```python
from build123d import *
from build123d.topology import SkipClean

# Parameters (mm, degrees)
SKETCH2_R           = 85
SKETCH2_R_2         = 20
BOSS_EXTRUDE1_DEPTH = 5
BOSS_EXTRUDE2_START = 155
SKETCH3_W           = 245
SKETCH3_H           = 230
SKETCH3_R           = 85
SKETCH3_W_2         = 265
SKETCH3_H_2         = 285
SKETCH3_R_2         = 20
BOSS_EXTRUDE2_DEPTH = 155
SKETCH4_W           = 33
SKETCH4_H           = 40
BOSS_EXTRUDE4_DEPTH = 70
SKETCH6_R           = 15
SKETCH6_W           = 63
SKETCH6_H           = 50
BOSS_EXTRUDE6_DEPTH = 22
SKETCH6_3_R         = 15
SKETCH6_3_R_2       = 6
BOSS_EXTRUDE7_DEPTH = 47
SKETCH6_4_R         = 6
BOSS_EXTRUDE8_DEPTH = 77
SKETCH2_4_R         = 85
CUT_EXTRUDE2_DEPTH  = 5


with BuildPart() as part:
    # Sketch2 → Boss-Extrude1 (new body)
    with BuildSketch(Plane.XY):
        Circle(SKETCH2_R)
        Circle(SKETCH2_R_2, mode=Mode.SUBTRACT)
    extrude(amount=BOSS_EXTRUDE1_DEPTH)

    # Sketch3 → Boss-Extrude2 (add)
    # profile 1 of 3: a face of its own
    with SkipClean():  # the faces are left unmerged after this step: merging them gives an invalid solid
        with BuildSketch(Plane(origin=(0, 0, 0), x_dir=(-1, 0, 0), z_dir=(0, 0, -1)).offset(BOSS_EXTRUDE2_START)):
            with Locations((-17.5, -20)):
                Rectangle(SKETCH3_W, SKETCH3_H)
            with Locations(Location((0, 0, 0), (0, 0, 180))):
                Circle(SKETCH3_R, mode=Mode.SUBTRACT)
        # profile 2 of 3: a face of its own
        with BuildSketch(Plane(origin=(0, 0, 0), x_dir=(-1, 0, 0), z_dir=(0, 0, -1)).offset(BOSS_EXTRUDE2_START)):
            with Locations((-272.5, 7.5)):
                Rectangle(SKETCH3_W_2, SKETCH3_H_2)
        # profile 3 of 3: a face of its own
        with BuildSketch(Plane(origin=(0, 0, 0), x_dir=(-1, 0, 0), z_dir=(0, 0, -1)).offset(BOSS_EXTRUDE2_START)):
            with Locations(Location((0, 0, 0), (0, 0, 180))):
                Circle(SKETCH3_R)
            Circle(SKETCH3_R_2, mode=Mode.SUBTRACT)
        extrude(amount=-BOSS_EXTRUDE2_DEPTH)

    # Sketch4 → Boss-Extrude4 (add)
    with SkipClean():  # the faces are left unmerged after this step: merging them gives an invalid solid
        with BuildSketch(Plane(origin=(0, 0, -155), x_dir=(-1, 0, 0), z_dir=(0, 0, -1))):
            with Locations((-83.5, 115)):
                Rectangle(SKETCH4_W, SKETCH4_H)
        extrude(amount=-BOSS_EXTRUDE4_DEPTH)

    # Sketch6 → Boss-Extrude6 (add)
    # profile 1 of 2: a face of its own
    with SkipClean():  # the faces are left unmerged after this step: merging them gives an invalid solid
        with BuildSketch(Plane.XZ.offset(135)):
            Polygon((-115, 50), (-115, 0), (-105, 0), (-52, 0), (-52, 50), align=None)
            with Locations(Location((-83.5, 25, 0), (0, 0, 270))):
                Circle(SKETCH6_R, mode=Mode.SUBTRACT)
        # profile 2 of 2: a face of its own
        with BuildSketch(Plane.XZ.offset(135)):
            with Locations((83.5, 25)):
                Rectangle(SKETCH6_W, SKETCH6_H)
            with Locations(Location((83.5, 25, 0), (0, 0, 270))):
                Circle(SKETCH6_R, mode=Mode.SUBTRACT)
        extrude(amount=-BOSS_EXTRUDE6_DEPTH)

    # Sketch6<3> → Boss-Extrude7 (add)
    # profile 1 of 2: a face of its own
    with SkipClean():  # the faces are left unmerged after this step: merging them gives an invalid solid
        with BuildSketch(Plane.XZ.offset(135)):
            with Locations(Location((-83.5, 25, 0), (0, 0, 270))):
                Circle(SKETCH6_3_R)
            with Locations(Location((-83.5, 25, 0), (0, 0, 270))):
                Circle(SKETCH6_3_R_2, mode=Mode.SUBTRACT)
        # profile 2 of 2: a face of its own
        with BuildSketch(Plane.XZ.offset(135)):
            with Locations(Location((83.5, 25, 0), (0, 0, 270))):
                Circle(SKETCH6_3_R)
            with Locations(Location((83.5, 25, 0), (0, 0, 270))):
                Circle(SKETCH6_3_R_2, mode=Mode.SUBTRACT)
        extrude(amount=-BOSS_EXTRUDE7_DEPTH)

    # Sketch6<4> → Boss-Extrude8 (add)
    with SkipClean():  # the faces are left unmerged after this step: merging them gives an invalid solid
        with BuildSketch(Plane.XZ.offset(135)):
            with Locations(Location((-83.5, 25, 0), (0, 0, 270))):
                Circle(SKETCH6_4_R)
            with Locations(Location((83.5, 25, 0), (0, 0, 270))):
                Circle(SKETCH6_4_R)
        extrude(amount=-BOSS_EXTRUDE8_DEPTH)

    # Sketch2<4> → Cut-Extrude2 (cut)
    with BuildSketch(Plane.XY):
        Circle(SKETCH2_4_R)
    extrude(amount=CUT_EXTRUDE2_DEPTH, mode=Mode.SUBTRACT)


solid = part.part
```
Here's how the part is built. I have some questions about the finished solid (model axes, mm). A direction names the side the tool comes from. Give positions to 0.01 mm unless a question says otherwise; leave off trailing zeros. Loops run counter-clockwise (first coordinate to the right, second up) from the corner with the lowest first, then second, coordinate; pieces in that order, holes last. Notation, with made-up numbers: M 36.25,-38 L 43.25,-38 A21 cw 43.25,0 Z; hole C 70,83 d7. An arc over 180 degrees is marked long. Use one line per item in the form item = value. Start each with the question number.
Q1. Will these pins go through, and if not, where does the flat tip stop? pin 1 Ø6 at (x, y) = (187, 96) entering from +Z; pin 2 Ø3 at (x, y) = (-108, -128.5) entering from -Z; pin 3 Ø16.5 at (x, y) = (83, 113.5) entering from +Z.
Q2. If we section it at B-B (y = 0): Write out the boundary of the cut face in (x, z).
Q3. If we section it at A-A (z = -126.5): Write out the boundary of the cut face in (x, y).
Q4. Thinking about a two-plate mould opening in Z: for faces 1 (the flat face through (154, 9, -155)), 2 (the flat face through (-83.3, -88, 18.5)), 3 (the flat face through (405, 6, -79)), 4 (the flat face through (84, 115, -85)), which applies, +Z half, -Z half, draft (parallel to the pull), parting line (faces both ways), or undercut?
Q5. If we section it at C-C (x = -83.5): Write out the boundary of the cut face in (y, z).
Q6. Which directions (+Z, -Z, +X, -X, +Y, -Y) give clear straight access to the entire face, cutting with the end or side of a thin tool? Please do faces 5 (the flat face through (84, 135, -120)), 6 (the flat face through (-83, -58, 25)), 7 (the flat face through (52, -124, 25)), 8 (the cylindrical face through (-98.143, -100.675, 28.252)), 9 (the flat face through (-110, -124, 0)).
Q7. I need wall thicknesses on line 1 along Y through (x, z) = (0, -31.5); line 2 along Z through (x, y) = (214.5, 71); line 3 along X through (y, z) = (48, -11.5). Which ranges of each line are inside material? Lowest first, please.
Q8. If we section it at D-D (z = 25): Write out the boundary of the cut face in (x, y).
Taken from the geometry:
q1.pin_1 = 0
q1.pin_2 = 0
q1.pin_3 = -85
q2.outline = M -105,-155 L -20,-155 L -20,0 L -105,0 Z; M 20,-155 L 405,-155 L 405,0 L 20,0 Z
q3.outline = M -105,-135 L 405,-135 L 405,150 L 140,150 L 140,95 L 100,95 L 100,135 L 67,135 L 67,95 L -105,95 Z; hole C 0,0 d40
q4.face_1 = -Z half
q4.face_2 = undercut
q4.face_3 = draft
q4.face_4 = +Z half
q5.outline = M -135,-155 L 95,-155 L 95,0 L -113,0 L -113,10 L -88,10 L -88,19 L -58,19 L -58,31 L -88,31 L -88,40 L -113,40 L -113,50 L -135,50 Z
q6.face_5 = +Z, -Z, -X, +Y
q6.face_6 = +Z, +X, -X, +Y
q6.face_7 = +Z, +Y, -Y
q6.face_8 = +Y
q6.face_9 = -Z, -X, +Y, -Y
q7.line_1 = -135 to -20, 20 to 95
q7.line_2 = -155 to 0
q7.line_3 = -105 to 405
q8.outline = M -115,-135 L -52,-135 L -52,-113 L -68.5,-113 L -68.5,-88 L -77.5,-88 L -77.5,-58 L -89.5,-58 L -89.5,-88 L -98.5,-88 L -98.5,-113 L -115,-113 Z; M 52,-135 L 115,-135 L 115,-113 L 98.5,-113 L 98.5,-88 L 89.5,-88 L 89.5,-58 L 77.5,-58 L 77.5,-88 L 68.5,-88 L 68.5,-113 L 52,-113 Z
